```python
from build123d import *

# Parameters (mm, degrees)
SKETCH_1_W           = 135
SKETCH_1_H           = 60
EXTRUDE_1_DEPTH      = 70
SKETCH_6_W           = 45
SKETCH_6_H           = 70
CUT_EXTRUDE_1_DEPTH  = 27.5
SKETCH_5_W           = 45
SKETCH_5_H           = 70
CUT_EXTRUDE_2_DEPTH  = 27.5
SKETCH_7_W           = 80
SKETCH_7_H           = 50
CUT_EXTRUDE_3_DEPTH  = 75
SKETCH_8_W           = 88
SKETCH_8_H           = 58
SKETCH_8_W_2         = 82
SKETCH_8_H_2         = 52
CUT_EXTRUDE_4_DEPTH  = 6
SKETCH_10_W          = 21.5
SKETCH_10_H          = 15
CUT_EXTRUDE_6_DEPTH  = 10
SKETCH_12_W          = 18.906228009
SKETCH_12_H          = 10
CUT_EXTRUDE_7_DEPTH  = 45
CUT_EXTRUDE_8_DEPTH  = 3
SKETCH_15_W          = 10
SKETCH_15_H          = 10
CUT_EXTRUDE_9_DEPTH  = 1
SKETCH_17_R          = 1.095275866
CUT_EXTRUDE_11_DEPTH = 7
SKETCH_18_W          = 5
SKETCH_18_H          = 5
SKETCH_18_R          = 1.05
EXTRUDE_2_DEPTH      = 5
SKETCH_19_W          = 90
SKETCH_19_H          = 60
EXTRUDE_3_DEPTH      = 2
SKETCH_20_R          = 4
CUT_EXTRUDE_12_DEPTH = 10
SKETCH_21_W          = 86
SKETCH_21_H          = 56
CUT_EXTRUDE_13_DEPTH = 63


with BuildPart() as part:
    # 草圖1 → 填料-伸長1 (new body)
    with BuildSketch(Plane.XY):
        with Locations((-8.008902174, -4.41011236)):
            Rectangle(SKETCH_1_W, SKETCH_1_H)
    extrude(amount=EXTRUDE_1_DEPTH)

    # 草圖6 → 除料-伸長1 (cut)
    with BuildSketch(Plane(origin=(0, 25.58988764, 0), x_dir=(1, 0, 0), z_dir=(0, 1, 0))):
        with Locations((36.991097826, -35)):
            Rectangle(SKETCH_6_W, SKETCH_6_H)
    extrude(amount=-CUT_EXTRUDE_1_DEPTH, mode=Mode.SUBTRACT)

    # 草圖5 → 除料-伸長2 (cut)
    with BuildSketch(Plane.XZ.offset(34.41011236)):
        with Locations((36.991097826, 35)):
            Rectangle(SKETCH_5_W, SKETCH_5_H)
    extrude(amount=-CUT_EXTRUDE_2_DEPTH, mode=Mode.SUBTRACT)

    # 草圖7 → 除料-伸長3 (cut)
    with BuildSketch(Plane.XY):
        with Locations((-30.508902174, -4.41011236)):
            Rectangle(SKETCH_7_W, SKETCH_7_H)
    extrude(amount=CUT_EXTRUDE_3_DEPTH, mode=Mode.SUBTRACT)

    # 草圖8 → 除料-伸長4 (cut)
    with BuildSketch(Plane(origin=(0, 0, 0), x_dir=(-1, 0, 0), z_dir=(0, 0, -1))):
        with Locations((30.508902174, -4.41011236)):
            Rectangle(SKETCH_8_W, SKETCH_8_H)
        with Locations((30.508902174, -4.41011236)):
            Rectangle(SKETCH_8_W_2, SKETCH_8_H_2, mode=Mode.SUBTRACT)
    extrude(amount=-CUT_EXTRUDE_4_DEPTH, mode=Mode.SUBTRACT)

    # 草圖10 → 除料-伸長6 (cut)
    with BuildSketch(Plane(origin=(0, -34.41011236, 0), x_dir=(-1, 0, 0), z_dir=(0, -1, 0))):
        with Locations((24.758902174, -19.5)):
            Rectangle(SKETCH_10_W, SKETCH_10_H)
    extrude(amount=-CUT_EXTRUDE_6_DEPTH, mode=Mode.SUBTRACT)

    # 草圖12 → 除料-伸長7 (cut)
    with BuildSketch(Plane(origin=(14.491097826, 0, 0), x_dir=(0, 0, -1), z_dir=(1, 0, 0))):
        with Locations((-60.546885996, -4.41011236)):
            Rectangle(SKETCH_12_W, SKETCH_12_H)
        with Locations((-9.453114004, -4.41011236)):
            Rectangle(SKETCH_12_W, SKETCH_12_H)
    extrude(amount=CUT_EXTRUDE_7_DEPTH, mode=Mode.SUBTRACT)

    # 草圖14 → 除料-伸長8 (cut)
    with BuildSketch(Plane(origin=(0, -6.91011236, 0), x_dir=(-1, 0, 0), z_dir=(0, -1, 0))):
        with BuildLine():
            Line((-38.126130034, -30.080170747), (-22.017914827, -33))
            ThreePointArc((-22.017914827, -33), (-20.017914827, -35), (-22.017914827, -37))
            Line((-22.017914827, -37), (-38.126130034, -39.919829253))
            ThreePointArc((-38.126130034, -39.919829253), (-39.017914827, -40), (-39.909699621, -39.919829253))
            Line((-39.909699621, -39.919829253), (-56.017914827, -37))
            ThreePointArc((-56.017914827, -37), (-58.017914827, -35), (-56.017914827, -33))
            Line((-56.017914827, -33), (-39.909699621, -30.080170747))
            ThreePointArc((-39.909699621, -30.080170747), (-39.017914827, -30), (-38.126130034, -30.080170747))
        make_face()
    extrude(amount=-CUT_EXTRUDE_8_DEPTH, mode=Mode.SUBTRACT)

    # 草圖15 → 除料-伸長9 (cut)
    with BuildSketch(Plane(origin=(0, -1.91011236, 0), x_dir=(1, 0, 0), z_dir=(0, 1, 0))):
        with Locations((39.491097826, -34.906228009)):
            Rectangle(SKETCH_15_W, SKETCH_15_H)
    extrude(amount=-CUT_EXTRUDE_9_DEPTH, mode=Mode.SUBTRACT)

    # 草圖17 → 除料-伸長11 (cut)
    with BuildSketch(Plane(origin=(0, -6.91011236, 0), x_dir=(-1, 0, 0), z_dir=(0, -1, 0))):
        with Locations((-39.017914827, -35)):
            Circle(SKETCH_17_R)
    extrude(amount=-CUT_EXTRUDE_11_DEPTH, mode=Mode.SUBTRACT)

    # 草圖18 → 填料-伸長2 (add)
    with BuildSketch(Plane.XY):
        with Locations((11.991097826, 28.08988764)):
            Rectangle(SKETCH_18_W, SKETCH_18_H)
        with Locations((11.991097826, 28.08988764)):
            Circle(SKETCH_18_R, mode=Mode.SUBTRACT)
        with Locations((-73.008902174, 28.08988764)):
            Rectangle(SKETCH_18_W, SKETCH_18_H)
        with Locations((-73.008902174, 28.08988764)):
            Circle(SKETCH_18_R, mode=Mode.SUBTRACT)
        with Locations((-73.008902174, -36.91011236)):
            Rectangle(SKETCH_18_W, SKETCH_18_H)
        with Locations((-73.008902174, -36.91011236)):
            Circle(SKETCH_18_R, mode=Mode.SUBTRACT)
        with Locations((11.991097826, -36.91011236)):
            Rectangle(SKETCH_18_W, SKETCH_18_H)
        with Locations((11.991097826, -36.91011236)):
            Circle(SKETCH_18_R, mode=Mode.SUBTRACT)
    extrude(amount=EXTRUDE_2_DEPTH)

    # 草圖19 → 填料-伸長3 (add)
    with BuildSketch(Plane.XY.offset(70)):
        with Locations((-30.508902174, -4.41011236)):
            Rectangle(SKETCH_19_W, SKETCH_19_H)
    extrude(amount=EXTRUDE_3_DEPTH)

    # 草圖20 → 除料-伸長12 (cut)
    with BuildSketch(Plane(origin=(14.491097826, 0, 0), x_dir=(0, 0, -1), z_dir=(1, 0, 0))):
        with Locations((-60, -21.41011236)):
            Circle(SKETCH_20_R)
        with Locations((-17, 12.58988764)):
            Circle(SKETCH_20_R)
    extrude(amount=-CUT_EXTRUDE_12_DEPTH, mode=Mode.SUBTRACT)

    # 草圖21 → 除料-伸長13 (cut)
    with BuildSketch(Plane(origin=(0, 0, 7), x_dir=(-1, 0, 0), z_dir=(0, 0, -1))):
        with Locations((30.508902174, -4.41011236)):
            Rectangle(SKETCH_21_W, SKETCH_21_H)
    extrude(amount=-CUT_EXTRUDE_13_DEPTH, mode=Mode.SUBTRACT)


solid = part.part
```
Here's how the part is built. I have some questions about the finished solid (model axes, mm). A direction names the side the tool comes from. Coordinates: 2 decimals unless noted, no trailing zeros. Loops run counter-clockwise (first coordinate to the right, second up) from the corner with the lowest first, then second, coordinate; pieces in that order, holes last. Notation, with made-up numbers: (89.5, 40) -> (131.5, 40) arc R25 ccw to (131.5, 77) -> close; hole circle Ø5 at (53, 49). An arc over 180 degrees is marked (long way). Return JSON: item names as keys, results as strings.
1) If we section it at B-B, the plane y = -11: Write out the boundary of the cut face in (x, z), then the cut area to 3 significant figures.
Results below:
{"outline": "(-75.51, 0) -> (-74.51, 0) -> (-74.51, 6) -> (-71.51, 6) -> (-71.51, 0) -> (-70.51, 0) -> (-70.51, 7) -> (-73.51, 7) -> (-73.51, 70) -> (12.49, 70) -> (12.49, 7) -> (9.49, 7) -> (9.49, 0) -> (10.49, 0) -> (10.49, 6) -> (13.49, 6) -> (13.49, 0) -> (14.49, 0) -> (14.49, 72) -> (-75.51, 72) -> close", "area": "466 mm²"}
2) I need wall thicknesses on line 1 (Y direction, x = -14.5, z = 60); line 2 (X direction, y = -27, z = 45.5); line 3 (X direction, y = -3, z = 35). Which ranges of each line are inside material? Lowest first, please. Write a range as from..to.
Results below:
{"line 1": "-34.41..-32.41, 23.59..25.59", "line 2": "-75.51..-73.51, 12.49..14.49", "line 3": "-75.51..-73.51, 12.49..37.92, 40.11..59.49"}
3) If we section it at A-A, the plane z = 48.5: Write out the boundary of the cut face in (x, y).
Results below:
{"outline": "(-75.51, -34.41) -> (14.49, -34.41) -> (14.49, -6.91) -> (59.49, -6.91) -> (59.49, -1.91) -> (14.49, -1.91) -> (14.49, 25.59) -> (-75.51, 25.59) -> close; hole (-73.51, -32.41) -> (12.49, -32.41) -> (12.49, 23.59) -> (-73.51, 23.59) -> close"}
4) If we section it at C-C, the plane z = 17: Write out the boundary of the cut face in (x, y), then the cut area to 3 significant figures.
Results below:
{"outline": "(-75.51, -34.41) -> (-35.51, -34.41) -> (-35.51, -32.41) -> (-73.51, -32.41) -> (-73.51, 23.59) -> (12.49, 23.59) -> (12.49, 16.59) -> (14.49, 16.59) -> (14.49, 25.59) -> (-75.51, 25.59) -> close; (-14.01, -34.41) -> (14.49, -34.41) -> (14.49, 8.59) -> (12.49, 8.59) -> (12.49, -32.41) -> (-14.01, -32.41) -> close", "area": "525 mm²"}
5) Will these pins go through, and if not, where does the flat tip stop? pin 1 (1.5 mm diameter, centred on x = 37, z = 47, fed in from -Y); pin 2 (11 mm diameter, centred on x = 38, z = 33.5, fed in from +Y); pin 3 (10 mm diameter, centred on x = 40, y = 1, fed in from +Z).
Results below:
{"pin 1": "y = -6.91", "pin 2": "y = -1.91", "pin 3": "z = 51.09"}
6) If we section it at D-D, the plane x = -9.5: Write out the boundary of the cut face in (y, z).
Results below:
{"outline": "(-34.41, 0) -> (-33.41, 0) -> (-33.41, 6) -> (-30.41, 6) -> (-30.41, 0) -> (-29.41, 0) -> (-29.41, 7) -> (-32.41, 7) -> (-32.41, 70) -> (23.59, 70) -> (23.59, 7) -> (20.59, 7) -> (20.59, 0) -> (21.59, 0) -> (21.59, 6) -> (24.59, 6) -> (24.59, 0) -> (25.59, 0) -> (25.59, 72) -> (-34.41, 72) -> close"}
7) Thinking about a two-plate mould opening in Y: for faces 5 (the face through (12, -39.41, 2)), 6 (the face through (48.08, -5.43, 31.56)), 7 (the face through (12.491, -5, 38)), which applies, +Y half, -Y half, draft (parallel to the pull), parting line (faces both ways), or undercut?
Results below:
{"face 5": "-Y half", "face 6": "draft", "face 7": "undercut"}
8) For faces 1 (the face through (-73.509, -5, 38)), 2 (the face through (37, -4, 51.094)), 3 (the face through (9.491, 28, 2)), 4 (the face through (10.8, -37.4, 5)), which set-ups out of +Z, -Z, +X, -X, +Y, -Y let a thin tool reach every point of the face, with its end or its side?
Results below:
{"face 1": "none", "face 2": "+Z, +X, +Y, -Y", "face 3": "+Z, -Z, +Y", "face 4": "+Z, +X, -X, -Y"}
